Check sheet for the modelled part. Datum: model origin and axes. Units: mm. A direction names the side the tool comes from. Round coordinates to 2 decimals unless told otherwise and drop trailing zeros. Loops run counter-clockwise (first coordinate to the right, second up) from the corner with the lowest first, then second, coordinate; pieces in that order, holes last. Notation, with made-up numbers: (58, -33.75) -> (78, -33.75) arc R6 ccw to (78, -23.75) -> close; hole circle Ø6 at (68, 78). An arc over 180 degrees is marked (long way). Return JSON: item names as keys, results as strings.
from build123d import *

# Parameters (mm, degrees)
F1_DEPTH = 12.5
F2_R     = 2.5
F3_DEPTH = 1.9009989591
F4_R     = 1.5
F5_DEPTH = 1.8999989591


with BuildPart() as f1:
    # F0 (on Front) → F1 (new body, symmetric)
    with BuildSketch(Plane.XZ):
        with BuildLine():
            Line((-50, 0), (0, 0))
            Line((0, 0), (0, 1.8999989591))
            Line((0, 1.8999989591), (-50, 1.8999989591))
            ThreePointArc((-50, 1.8999989591), (-52.309699793, 3.4432910207), (-51.767767689, 6.167767689))
            Line((-51.767767689, 6.167767689), (-34.0900981594, 23.8454372187))
            Line((-34.0900981594, 23.8454372187), (-35.4336003076, 25.1889393669))
            Line((-35.4336003076, 25.1889393669), (-53.1112698372, 7.5112698372))
            ThreePointArc((-53.1112698372, 7.5112698372), (-54.065069943, 2.7161928976), (-50, 0))
        make_face()
    extrude(amount=F1_DEPTH, both=True)

    # F2 (on face) → F3 (cut, through all)
    with BuildSketch(Plane.XY.offset(1.8999989591)):
        with Locations((-32, 0)):
            Circle(F2_R)
        with BuildLine():
            Line((0, 12.5), (-4.5, 12.5))
            ThreePointArc((-4.5, 12.5), (-1.3180194847, 11.1819805153), (0, 8))
            Line((0, 8), (0, 12.5))
        make_face()
        with BuildLine():
            Line((0, -12.5), (0, -8))
            ThreePointArc((0, -8), (-1.3180194847, -11.1819805153), (-4.5, -12.5))
            Line((-4.5, -12.5), (0, -12.5))
        make_face()
        with BuildLine():
            Line((-7, 2.5), (-22, 2.5))
            ThreePointArc((-22, 2.5), (-24.5, 0), (-22, -2.5))
            Line((-22, -2.5), (-7, -2.5))
            ThreePointArc((-7, -2.5), (-4.5, 0), (-7, 2.5))
        make_face()
    extrude(amount=-F3_DEPTH, mode=Mode.SUBTRACT)

    # F4 (on face) → F5 (cut, through all)
    with BuildSketch(Plane(origin=(-30.3112698372, 0, 30.3112698372), x_dir=(0, -1, 0), z_dir=(-0.7071067812, 0, 0.7071067812))):
        with Locations((-8, -14.7440692221)):
            Circle(F4_R)
        with BuildLine():
            Line((-12.5, -7.2440692221), (-12.5, -12.2440692221))
            ThreePointArc((-12.5, -12.2440692221), (-11.0355339059, -8.7085353162), (-7.5, -7.2440692221))
            Line((-7.5, -7.2440692221), (-12.5, -7.2440692221))
        make_face()
        with Locations((8, -14.7440692221)):
            Circle(F4_R)
        with BuildLine():
            ThreePointArc((7.5, -7.2440692221), (11.0355339059, -8.7085353162), (12.5, -12.2440692221))
            Line((12.5, -12.2440692221), (12.5, -7.2440692221))
            Line((12.5, -7.2440692221), (7.5, -7.2440692221))
        make_face()
    extrude(amount=-F5_DEPTH, mode=Mode.SUBTRACT)


solid = f1.part
Q1. Material ranges on line 1 (Y direction, x = -32, z = 0.4); line 2 (Z direction, x = -17.5, y = -10); line 3 (Z direction, x = -38, y = -4), recorded low to high.
Results list:
{"line 1": "-12.5 to -2.5, 2.5 to 12.5", "line 2": "0 to 1.9", "line 3": "0 to 1.9, 19.94 to 22.62"}
Q2. Tool access check on faces 4 (the flat face through (-25, 0, 1.9)), 5 (the flat face through (-15, -2.5, 1)), 6 (the cylindrical face through (-1.353, 11.217, 0.963)). Record the directions out of +Z, -Z, +X, -X, +Y, -Y that give a thin tool (end or side, any length) a straight path to the whole face; none if there is none.
Results list:
{"face 4": "+X, +Y, -Y", "face 5": "+Z, -Z", "face 6": "+Z, -Z, +X, +Y"}
Q3. Section check D-D (x = -45). Record the boundary of the cut face in (y, z).
Results list:
{"outline": "(-12.5, 0) -> (12.5, 0) -> (12.5, 1.9) -> (-12.5, 1.9) -> close; (-12.5, 12.94) -> (12.5, 12.94) -> (12.5, 15.62) -> (-12.5, 15.62) -> close"}
Q4. Draft check along Z on faces 1 (the cylindrical face through (-35.834, 11.074, 23.463)), 2 (the flat face through (0, 0, 1)), 3 (the flat face through (-43.053, -0.175, 14.883)). Enter one of: released by +Z, released by -Z, zero draft, split by the parting line, or undercut.
Results list:
{"face 1": "released by +Z", "face 2": "zero draft", "face 3": "undercut"}
Q5. Section check B-B (x = -18). Record the boundary of the cut face in (y, z).
Results list:
{"outline": "(-12.5, 0) -> (-2.5, 0) -> (-2.5, 1.9) -> (-12.5, 1.9) -> close; (2.5, 0) -> (12.5, 0) -> (12.5, 1.9) -> (2.5, 1.9) -> close"}
Q6. Go/stop test with flat-tipped pins: pin 1 (2 mm diameter, centred on x = -36, y = 9, fed in from -Z); pin 2 (10 mm diameter, centred on y = 8, z = 20.5, fed in from -X); pin 3 (4 mm diameter, centred on y = 7.5, z = 12, fed in from +X); pin 4 (4 mm diameter, centred on y = -2, z = 7, fed in from +X). Record where each tip stops, or that it passes through.
Results list:
{"pin 1": "z = 0", "pin 2": "x = -45.12", "pin 3": "x = -43.94", "pin 4": "x = -48.94"}
Q7. Section check C-C (y = 5.25). Record the boundary of the cut face in (x, z).
Results list:
{"outline": "(-53.11, 7.51) arc R4.4 ccw to (-50, 0) -> (0, 0) -> (0, 1.9) -> (-50, 1.9) arc R2.5 cw to (-51.77, 6.17) -> (-34.09, 23.85) -> (-35.43, 25.19) -> close"}
Q8. Section check A-A (y = 0). Record the boundary of the cut face in (x, z), then the cut area to 3 significant figures.
Results list:
{"outline": "(-53.11, 7.51) arc R4.4 ccw to (-50, 0) -> (-34.5, 0) -> (-34.5, 1.9) -> (-50, 1.9) arc R2.5 cw to (-51.77, 6.17) -> (-34.09, 23.85) -> (-35.43, 25.19) -> close; (-29.5, 0) -> (-24.5, 0) -> (-24.5, 1.9) -> (-29.5, 1.9) -> close; (-4.5, 0) -> (0, 0) -> (0, 1.9) -> (-4.5, 1.9) -> close", "area": "110 mm^2"}
